from build123d import *

# Parameters (mm, degrees)
BASE_FLANGE1_DEPTH         = 1
SKETCHED_START             = 31
SKETCHED_BEND1_DEPTH       = 178
SKETCHED_BEND1_2_DEPTH     = 98
SKETCHED_BEND1_3_DEPTH     = 178
SKETCHED_BEND1_4_OUTLINE_W = 98
SKETCHED_BEND1_4_OUTLINE_H = 1
SKETCHED_BEND1_4_DEPTH     = 29.234623369
SKETCHED_START_2           = 210.765376631
SKETCHED_BEND1_5_OUTLINE_W = 98
SKETCHED_BEND1_5_OUTLINE_H = 1
SKETCHED_BEND1_5_DEPTH     = 29.234623369
SKETCHED_BEND1_6_DEPTH     = 98
SKETCHED_BEND1_7_OUTLINE_W = 178
SKETCHED_BEND1_7_OUTLINE_H = 1
SKETCHED_BEND1_7_DEPTH     = 29.234623369
SKETCHED_START_3           = 130.765376631
SKETCHED_BEND1_8_OUTLINE_W = 178
SKETCHED_BEND1_8_OUTLINE_H = 1
SKETCHED_BEND1_8_DEPTH     = 29.234623369


# Read off the part's stored shape, not the designer's step: Sketched Bend1
# Sheet-metal steps are written as plain solids
with BuildPart() as part:
    # Sketch1 → Base-Flange1 (new body)
    with BuildSketch(Plane.XY):
        Polygon((0, 209), (31, 209), (31, 240), (129, 240), (129, 209), (160, 209), (160, 31), (129, 31), (129, 0), (31, 0), (31, 31), (0, 31), align=None)
    extrude(amount=-BASE_FLANGE1_DEPTH)

    # Sketched Bend1 outline → Sketched Bend1 (add)
    with BuildSketch(Plane(origin=(0, 0, 0), x_dir=(1, 0, 0), z_dir=(0, 1, 0)).offset(SKETCHED_START)):
        with BuildLine():
            Line((29.234623369, -0.7366), (29.234623369, -29.765376631))
            Line((29.234623369, -29.765376631), (30.234623369, -29.765376631))
            Line((30.234623369, -29.765376631), (30.234623369, -0.7366))
            ThreePointArc((30.234623369, -0.7366), (30.450368514, -0.215745145), (30.971223369, 0))
            Line((30.971223369, 0), (29.398582279, 0))
            ThreePointArc((29.398582279, 0), (29.276108612, -0.359286442), (29.234623369, -0.7366))
        make_face()
        with BuildLine():
            Line((130.601417721, 0), (129.028776631, 0))
            ThreePointArc((129.028776631, 0), (129.549631486, -0.215745145), (129.765376631, -0.7366))
            Line((129.765376631, -0.7366), (129.765376631, -29.765376631))
            Line((129.765376631, -29.765376631), (130.765376631, -29.765376631))
            Line((130.765376631, -29.765376631), (130.765376631, -0.7366))
            ThreePointArc((130.765376631, -0.7366), (130.723891388, -0.359286442), (130.601417721, 0))
        make_face()
    extrude(amount=SKETCHED_BEND1_DEPTH)

    # Sketched Bend1 2 outline → Sketched Bend1 2 (add)
    with BuildSketch(Plane.YZ.offset(SKETCHED_START)):
        with BuildLine():
            Line((209.028776631, 0), (210.601417721, 0))
            ThreePointArc((210.601417721, 0), (210.723891388, 0.359286442), (210.765376631, 0.7366))
            Line((210.765376631, 0.7366), (210.765376631, 29.765376631))
            Line((210.765376631, 29.765376631), (209.765376631, 29.765376631))
            Line((209.765376631, 29.765376631), (209.765376631, 0.7366))
            ThreePointArc((209.765376631, 0.7366), (209.549631486, 0.215745145), (209.028776631, 0))
        make_face()
        with BuildLine():
            ThreePointArc((29.234623369, 0.7366), (29.276108612, 0.359286442), (29.398582279, 0))
            Line((29.398582279, 0), (30.971223369, 0))
            ThreePointArc((30.971223369, 0), (30.450368514, 0.215745145), (30.234623369, 0.7366))
            Line((30.234623369, 0.7366), (30.234623369, 29.765376631))
            Line((30.234623369, 29.765376631), (29.234623369, 29.765376631))
            Line((29.234623369, 29.765376631), (29.234623369, 0.7366))
        make_face()
    extrude(amount=SKETCHED_BEND1_2_DEPTH)

    # Sketched Bend1 3 outline → Sketched Bend1 3 (cut)
    with BuildSketch(Plane(origin=(0, 0, 0), x_dir=(1, 0, 0), z_dir=(0, 1, 0)).offset(SKETCHED_START)):
        with BuildLine():
            Line((0, 0), (29.398582279, 0))
            ThreePointArc((29.398582279, 0), (30.039397205, 0.728828115), (30.971223369, 1))
            Line((30.971223369, 1), (0, 1))
            Line((0, 1), (0, 0))
        make_face()
        with BuildLine():
            Line((160, 1), (129.028776631, 1))
            ThreePointArc((129.028776631, 1), (129.960602795, 0.728828115), (130.601417721, 0))
            Line((130.601417721, 0), (160, 0))
            Line((160, 0), (160, 1))
        make_face()
    extrude(amount=SKETCHED_BEND1_3_DEPTH, mode=Mode.SUBTRACT)

    # Sketched Bend1 4 outline → Sketched Bend1 4 (cut)
    with BuildSketch(Plane(origin=(0, 0, 0), x_dir=(1, 0, 0), z_dir=(0, 1, 0))):
        with Locations((80, 0.5)):
            Rectangle(SKETCHED_BEND1_4_OUTLINE_W, SKETCHED_BEND1_4_OUTLINE_H)
    extrude(amount=SKETCHED_BEND1_4_DEPTH, mode=Mode.SUBTRACT)

    # Sketched Bend1 5 outline → Sketched Bend1 5 (cut)
    with BuildSketch(Plane(origin=(0, 0, 0), x_dir=(1, 0, 0), z_dir=(0, 1, 0)).offset(SKETCHED_START_2)):
        with Locations((80, 0.5)):
            Rectangle(SKETCHED_BEND1_5_OUTLINE_W, SKETCHED_BEND1_5_OUTLINE_H)
    extrude(amount=SKETCHED_BEND1_5_DEPTH, mode=Mode.SUBTRACT)

    # Sketched Bend1 6 outline → Sketched Bend1 6 (cut)
    with BuildSketch(Plane.YZ.offset(SKETCHED_START)):
        with BuildLine():
            ThreePointArc((210.601417721, 0), (209.960602795, -0.728828115), (209.028776631, -1))
            Line((209.028776631, -1), (240, -1))
            Line((240, -1), (240, 0))
            Line((240, 0), (210.601417721, 0))
        make_face()
        with BuildLine():
            Line((0, -1), (30.971223369, -1))
            ThreePointArc((30.971223369, -1), (30.039397205, -0.728828115), (29.398582279, 0))
            Line((29.398582279, 0), (0, 0))
            Line((0, 0), (0, -1))
        make_face()
    extrude(amount=SKETCHED_BEND1_6_DEPTH, mode=Mode.SUBTRACT)

    # Sketched Bend1 7 outline → Sketched Bend1 7 (cut)
    with BuildSketch(Plane.YZ):
        with Locations((120, -0.5)):
            Rectangle(SKETCHED_BEND1_7_OUTLINE_W, SKETCHED_BEND1_7_OUTLINE_H)
    extrude(amount=SKETCHED_BEND1_7_DEPTH, mode=Mode.SUBTRACT)

    # Sketched Bend1 8 outline → Sketched Bend1 8 (cut)
    with BuildSketch(Plane.YZ.offset(SKETCHED_START_3)):
        with Locations((120, -0.5)):
            Rectangle(SKETCHED_BEND1_8_OUTLINE_W, SKETCHED_BEND1_8_OUTLINE_H)
    extrude(amount=SKETCHED_BEND1_8_DEPTH, mode=Mode.SUBTRACT)


solid = part.part
Geometry: final body of the model. Coordinates: model frame, mm. A direction names the side the tool comes from. Coordinates: 2 decimals unless noted, no trailing zeros. Write each loop counter-clockwise with the first axis right and the second up, starting at its lowest first coordinate (ties: lowest second). Pieces come first, ordered by that corner, then holes. Notation, with made-up numbers: (31, -5) - (63, -5) arc R33 ccw to (63, 28) - close; hole circle Ø5 at (5, 62). An arc over 180 degrees is marked (long way). Return JSON: item names as keys, results as strings.
Item 1: Pull-direction query (X, two-part tool) for faces 1 (the face through (81, 121, 0)), 2 (the face through (130.765, 119, 15)), 3 (the face through (79, 29.235, 15)); classes: +X half, -X half, draft (parallel to the pull), parting line (faces both ways), or undercut.
Completed:
{"face 1": "undercut", "face 2": "+X half", "face 3": "draft"}
Item 2: Reachability of faces 4 (the face through (81, 121, -1)), 5 (the face through (30.235, 119, 15)), 6 (the face through (79, 209.765, 15)) from +Z, -Z, +X, -X, +Y, -Y: full face, straight path, thin tool, end or side. Return the list, or none.
Completed:
{"face 4": "-Z, +X, -X, +Y, -Y", "face 5": "+Z, +Y, -Y", "face 6": "+Z, +X, -X"}
Item 3: Section query B-B (y = 113). Output: boundary loops of the cut face in (x, z), and give its area (3 significant figures).
Completed:
{"outline": "(29.23, 0.74) arc R1.74 ccw to (30.97, -1) - (129.03, -1) arc R1.74 ccw to (130.77, 0.74) - (130.77, 29.77) - (129.77, 29.77) - (129.77, 0.74) arc R0.74 cw to (129.03, 0) - (30.97, 0) arc R0.74 cw to (30.23, 0.74) - (30.23, 29.77) - (29.23, 29.77) - close", "area": "160 mm2"}
Item 4: Section query C-C (x = 115). Output: boundary loops of the cut face in (y, z), and give its area (3 significant figures).
Completed:
{"outline": "(29.23, 0.74) arc R1.74 ccw to (30.97, -1) - (209.03, -1) arc R1.74 ccw to (210.77, 0.74) - (210.77, 29.77) - (209.77, 29.77) - (209.77, 0.74) arc R0.74 cw to (209.03, 0) - (30.97, 0) arc R0.74 cw to (30.23, 0.74) - (30.23, 29.77) - (29.23, 29.77) - close", "area": "240 mm2"}
Item 5: Section query A-A (z = 20). Output: boundary loops of the cut face in (x, y).
Completed:
{"outline": "(29.23, 31) - (30.23, 31) - (30.23, 209) - (29.23, 209) - close; (31, 29.23) - (129, 29.23) - (129, 30.23) - (31, 30.23) - close; (31, 209.77) - (129, 209.77) - (129, 210.77) - (31, 210.77) - close; (129.77, 31) - (130.77, 31) - (130.77, 209) - (129.77, 209) - close"}
Item 6: Line query: L1, parallel to X at y = 203, z = 12.5; L2, parallel to Y at x = 74, z = 15; L3, parallel to Y at x = 90, z = 0.5. Output: solid intervals per line, ascending.
Completed:
{"L1": "x = 29.23 to 30.23, 129.77 to 130.77", "L2": "y = 29.23 to 30.23, 209.77 to 210.77", "L3": "y = 29.25 to 30.27, 209.73 to 210.75"}
Item 7: Pin query (flat end, axial travel): pin 1 Ø1.9 at (x, z) = (30, 14) entering from +Y; pin 2 Ø0.9 at (x, z) = (129.5, 7) entering from -Y; pin 3 Ø6 at (x, y) = (98, 120.5) entering from +Z. Return the tip coordinate at first contact, or that it passes through.
Completed:
{"pin 1": "stops at y = 209", "pin 2": "stops at y = 31", "pin 3": "stops at z = 0"}
